Autodesk Inventor part; units mm, degrees
ref_plane "YZ Plane" through (0, 0, 0) normal (1, 0, 0) x (0, 1, 0)
ref_plane "XZ Plane" through (0, 0, 0) normal (0, 1, 0) x (-1, 0, 0)
ref_plane "XY Plane" through (0, 0, 0) normal (0, 0, 1) x (1, 0, 0)
sketch "Sketch1" plane through (0, 0, 0) normal (0, 1, 0) x (-1, 0, 0)
  line L0 (-35, 32.5) -> (35, 32.5)
  line L1 (35, 32.5) -> (35, -32.5)
  line L2 (35, -32.5) -> (-35, -32.5)
  line L3 (-35, -32.5) -> (-35, 32.5)
  line L4 (-35, 32.5) -> (35, -32.5) construction
  line L5 (35, 32.5) -> (-35, -32.5) construction
  line L6 (-35, 22.5) -> (35, 22.5)
  line L7 (35, 22.5) -> (35, -22.5)
  line L8 (35, -22.5) -> (-35, -22.5)
  line L9 (-35, -22.5) -> (-35, 22.5)
  line L10 (-35, 22.5) -> (35, -22.5) construction
  line L11 (35, 22.5) -> (-35, -22.5) construction
  point P0 (0, 0)
  dimension "d0" = 70
  dimension "d1" = 65
  dimension "d2" = 10
extrude "Extrusion1" add sketch "Sketch1" along normal blind 10
sketch "Sketch2" plane through (0, 0, 0) normal (0, -1, 0) x (1, 0, 0)
  line L0 (35, 32.5) -> (35, -32.5)
  line L1 (-35, 32.5) -> (35, 32.5)
  line L2 (-35, -32.5) -> (-35, 32.5)
  line L3 (35, -32.5) -> (-35, -32.5)
  line L4 (-35, 22.5) -> (35, 22.5)
  line L5 (35, 22.5) -> (35, -22.5)
  line L6 (35, -22.5) -> (-35, -22.5)
  line L7 (-35, -22.5) -> (-35, 22.5)
  line L8 (-35, 22.5) -> (35, -22.5) construction
  line L9 (35, 22.5) -> (-35, -22.5) construction
  line L10 (35, 32.5) -> (35, -32.5)
  line L11 (-35, -22.5) -> (35, -32.5) construction
  line L12 (0, -27.5) -> (29, -27.5) construction
  point P0 (0, 0)
  dimension "d5" = 10
  dimension "d6" = 6
hole "Hole1" at (29, 0, -27.5) direction (0, 1, 0) diameter 4.2 end through all counterbore diameter 8 counterbore depth 4
mirror "Mirror1" about plane through (0, 0, 0) normal (1, 0, 0) of "Hole1"
mirror "Mirror2" about plane through (0, 0, 0) normal (0, 0, 1) of "Hole1", "Mirror1"
fillet "Fillet1" radius 2 4 edges at (35, 5, 32.5) (-35, 5, 32.5) (-35, 5, -32.5) (35, 5, -32.5)
sketch "Sketch3" plane through (0, 0, 0) normal (0, -1, 0) x (1, 0, 0)
  arc A0 (33, -32.5) -> (35, -30.5) centre (33, -30.5) ccw
  line L0 (35, 30.5) -> (35, -30.5)
  arc A1 (35, 30.5) -> (33, 32.5) centre (33, 30.5) ccw
  line L1 (-33, 32.5) -> (33, 32.5)
  arc A2 (-33, 32.5) -> (-35, 30.5) centre (-33, 30.5) ccw
  line L2 (-35, -30.5) -> (-35, 30.5)
  arc A3 (-35, -30.5) -> (-33, -32.5) centre (-33, -30.5) ccw
  line L3 (33, -32.5) -> (-33, -32.5)
  circle A4 centre (-29, 27.5) radius 4
  circle A5 centre (29, 27.5) radius 4
  circle A6 centre (-29, -27.5) radius 4
  circle A7 centre (29, -27.5) radius 4
  circle A8 centre (29, 27.5) radius 2.1
  circle A9 centre (-29, 27.5) radius 4
  line L4 (29, 27.5) -> (-29, 27.5)
  circle A10 centre (29, -27.5) radius 2.1
  line L5 (29, -27.5) -> (-29, -27.5)
  point P0 (0, 0)
  point P1 (0, 27.5)
  point P2 (0, -27.5)
hole "Hole2" at (0, 0, 27.5) at (0, 0, -27.5) direction (0, 1, 0) diameter 2.8 end through all
properties part number "23_Nap_hop_so_ngang" material "Stainless Steel, Austenitic"
Here's how the part is built. I have some questions about the finished solid (model axes, mm). A direction names the side the tool comes from. Give positions to 0.01 mm unless a question says otherwise; leave off trailing zeros. Order: outer loops, then holes, each group sorted by start corner. A loop starts at its lowest first (then second) coordinate and runs counter-clockwise, first axis right, second up. Notation, with made-up numbers: M 89.5,-16 L 132.5,-16 A16 ccw 132.5,3 Z; hole C 23.5,75 d1. An arc over 180 degrees is marked long. Use a Markdown table: item, result. Add a question column.
1. Suppose I cut it at C-C (x = 0). List the corners of the cut face in (y, z) for me, and give its area (3 significant figures).
2. I need wall thicknesses on probe 1 along X at (y, z) = (6, -27.5); probe 2 along X at (y, z) = (0.95, 27.5); probe 3 along Z at (x, y) = (29, 8.55). Which ranges of each line are inside material? Lowest first, please. Write a range as from..to.
3. Suppose I cut it at D-D (x = -29). List the corners of the cut face in (y, z) for me, and give its area (3 significant figures).
4. On a 3-axis mill with a long thin cutter (end or side, diameter ignored), from which of +Z, -Z, +X, -X, +Y, -Y can I reach the whole of each face in a straight line? I mean faces 1 (the cylindrical face through (-34.4, 5.07, -31.93)), 2 (the flat face through (-31, 4, -26)). Say none if no direction works.
5. Suppose I cut it at B-B (z = -27.5). List the corners of the cut face in (x, y) for me, and give its area (3 significant figures).
6. For pin 1 Ø9 at (x, z) = (27, -27.5) entering from -Y; pin 2 Ø2.5 at (x, z) = (-27.5, -26.5) entering from -Y, each with a flat end and sliding along its axis, tell me the tip position at first contact or that it passes through.
7. Suppose I cut it at A-A (y = 8.75). List the corners of the cut face in (x, z) for me, and give its area (3 significant figures).
8. If we mould it in two halves opening along X, with no side actions, what happens to faces 3 (the flat face through (31, 4, -29)), 4 (the cylindrical face through (34.4, 5.07, 31.93)), 5 (the cylindrical face through (27.722, 7.042, 25.834)), 6 (the flat face through (0, 5, -32.5))? For each: +X half, -X half, draft (parallel to the pull), parting line (faces both ways), or undercut.
Results list:
| question | item | result |
|---|---|---|
| 1 | outline | M 0,-32.5 L 10,-32.5 L 10,-28.9 L 0,-28.9 Z; M 0,-26.1 L 10,-26.1 L 10,26.1 L 0,26.1 Z; M 0,28.9 L 10,28.9 L 10,32.5 L 0,32.5 Z |
| 1 | area | 594 mm² |
| 2 | probe 1 | x = -35..-31.1, -26.9..-1.4, 1.4..26.9, 31.1..35 |
| 2 | probe 2 | x = -35..-33, -25..-1.4, 1.4..25, 33..35 |
| 2 | probe 3 | z = -32.5..-29.6, -25.4..25.4, 29.6..32.5 |
| 3 | outline | M 0,-32.5 L 10,-32.5 L 10,-29.6 L 4,-29.6 L 4,-31.5 L 0,-31.5 Z; M 0,-23.5 L 4,-23.5 L 4,-25.4 L 10,-25.4 L 10,25.4 L 4,25.4 L 4,23.5 L 0,23.5 Z; M 0,31.5 L 4,31.5 L 4,29.6 L 10,29.6 L 10,32.5 L 0,32.5 Z |
| 3 | area | 536 mm² |
| 4 | face 1 | -Z, -X, +Y, -Y |
| 4 | face 2 | -Y |
| 5 | outline | M -35,0 L -33,0 L -33,4 L -31.1,4 L -31.1,10 L -35,10 Z; M -26.9,4 L -25,4 L -25,0 L -1.4,0 L -1.4,10 L -26.9,10 Z; M 1.4,0 L 25,0 L 25,4 L 26.9,4 L 26.9,10 L 1.4,10 Z; M 31.1,4 L 33,4 L 33,0 L 35,0 L 35,10 L 31.1,10 Z |
| 5 | area | 558 mm² |
| 6 | pin 1 | stops at y = 0 |
| 6 | pin 2 | stops at y = 4 |
| 7 | outline | M -35,-30.5 A2 ccw -33,-32.5 L 33,-32.5 A2 ccw 35,-30.5 L 35,30.5 A2 ccw 33,32.5 L -33,32.5 A2 ccw -35,30.5 Z; hole C -29,-27.5 d4.2; hole C -29,27.5 d4.2; hole C 0,-27.5 d2.8; hole C 0,27.5 d2.8; hole C 29,-27.5 d4.2; hole C 29,27.5 d4.2 |
| 7 | area | 4,480 mm² |
| 8 | face 3 | undercut |
| 8 | face 4 | +X half |
| 8 | face 5 | undercut |
| 8 | face 6 | draft |
